Geometry check sheet. Reference: the model listing, model coordinates, mm. A direction names the side the tool comes from. Give positions to 0.01 mm unless a question says otherwise; leave off trailing zeros. Order: outer loops, then holes, each group sorted by start corner. A loop starts at its lowest first (then second) coordinate and runs counter-clockwise, first axis right, second up.
from build123d import *

# Parameters (mm, degrees)
SKETCH2_R           = 3.175
BOSS_EXTRUDE1_DEPTH = 1.57


with BuildPart() as part:
    # Sketch2 → Boss-Extrude1 (new body)
    with BuildSketch(Plane.XY.offset(5)):
        with BuildLine():
            Line((-16.920508995, 36.97485167), (-16.920508995, -35.724508995))
            Line((-16.920508995, -35.724508995), (-10.670508995, -35.724508995))
            Line((-10.670508995, -35.724508995), (-10.670508995, -24.224508995))
            Line((-10.670508995, -24.224508995), (10.670508995, -24.224508995))
            Line((10.670508995, -24.224508995), (10.670508995, -35.724508995))
            Line((10.670508995, -35.724508995), (16.920508995, -35.724508995))
            Line((16.920508995, -35.724508995), (16.920508995, 36.97485167))
            add(Edge.make_bspline(
                [(16.17485167, 37.720508995), (16.268017422, 37.720508995), (16.450238191, 37.688464247), (16.71855323, 37.51855323), (16.888464247, 37.250238191), (16.920508995, 37.068017422), (16.920508995, 36.97485167)],
                knots=[0, 0, 0, 0, 0.25, 0.5, 0.75, 1, 1, 1, 1], degree=3))
            Line((16.17485167, 37.720508995), (14.25, 37.720508995))
            ThreePointArc((14.25, 37.720508995), (11.718917637, 38.768917637), (10.670508995, 41.3))
            Line((10.670508995, 41.3), (10.670508995, 43.22485167))
            add(Edge.make_bspline(
                [(9.92485167, 43.970508995), (10.018017422, 43.970508995), (10.200238191, 43.938464247), (10.46855323, 43.76855323), (10.638464247, 43.500238191), (10.670508995, 43.318017422), (10.670508995, 43.22485167)],
                knots=[0, 0, 0, 0, 0.25, 0.5, 0.75, 1, 1, 1, 1], degree=3))
            Line((9.92485167, 43.970508995), (-9.92485167, 43.970508995))
            add(Edge.make_bspline(
                [(-10.670508995, 43.22485167), (-10.670508995, 43.318017422), (-10.638464247, 43.500238191), (-10.46855323, 43.76855323), (-10.200238191, 43.938464247), (-10.018017422, 43.970508995), (-9.92485167, 43.970508995)],
                knots=[0, 0, 0, 0, 0.25, 0.5, 0.75, 1, 1, 1, 1], degree=3))
            Line((-10.670508995, 43.22485167), (-10.670508995, 41.3))
            ThreePointArc((-10.670508995, 41.3), (-11.718917637, 38.768917637), (-14.25, 37.720508995))
            Line((-14.25, 37.720508995), (-16.17485167, 37.720508995))
            add(Edge.make_bspline(
                [(-16.920508995, 36.97485167), (-16.920508995, 37.068017422), (-16.888464247, 37.250238191), (-16.71855323, 37.51855323), (-16.450238191, 37.688464247), (-16.268017422, 37.720508995), (-16.17485167, 37.720508995)],
                knots=[0, 0, 0, 0, 0.25, 0.5, 0.75, 1, 1, 1, 1], degree=3))
        make_face()
        with Locations((0, -16.224508995)):
            Circle(SKETCH2_R, mode=Mode.SUBTRACT)
    extrude(amount=BOSS_EXTRUDE1_DEPTH)


solid = part.part
Item 1: Sectioned sample at B-B (y = -25.5). Enter the section's corners in (x, z).
Reported:
outline: (-16.92, 5) - (-10.67, 5) - (-10.67, 6.57) - (-16.92, 6.57) - close; (10.67, 5) - (16.92, 5) - (16.92, 6.57) - (10.67, 6.57) - close
Item 2: Sectioned sample at C-C (x = -12). Enter the section's corners in (y, z), and give its area (3 significant figures).
Reported:
outline: (-35.72, 5) - (38.52, 5) - (38.52, 6.57) - (-35.72, 6.57) - close
area: 117 mm2
Item 3: Sectioned sample at D-D (y = 39.5). Enter the section's corners in (x, z), and give its area (3 significant figures).
Reported:
outline: (-11.16, 5) - (11.16, 5) - (11.16, 6.57) - (-11.16, 6.57) - close
area: 35.0 mm2
Item 4: Gauge pin test, flat ends, axial feed: pin 1 (7.5 mm diameter, centred on x = 0, y = -16.22, fed in from +Z); pin 2 (0.8 mm diameter, centred on x = 0.5, z = 5.5, fed in from -Y); pin 3 (0.5 mm diameter, centred on x = 15, z = 5.5, fed in from +Y); pin 4 (0.8 mm diameter, centred on y = 42.5, z = 5.5, fed in from -X). Record the tip position at first contact, or that the pin passes through.
Reported:
pin 1: stops at z = 6.57
pin 2: stops at y = -24.22
pin 3: stops at y = 37.72
pin 4: stops at x = -10.67
Item 5: Set-up check for faces 4 (the flat face through (10.671, -30, 6)), 5 (the flat face through (16.921, 0, 6)), 6 (the flat face through (-10.671, 42, 6)), 7 (the flat face through (10.671, 42, 6)), 8 (the flat face through (0, 43.971, 6)): record each of +Z, -Z, +X, -X, +Y, -Y from which the full face is reachable in a straight line by a thin tool's end or side.
Reported:
face 4: +Z, -Z, -Y
face 5: +Z, -Z, +X, +Y, -Y
face 6: +Z, -Z, -X, +Y
face 7: +Z, -Z, +X, +Y
face 8: +Z, -Z, +X, -X, +Y
Item 6: Scan lines: L1, parallel to Y at x = 0, z = 5.45; L2, parallel to Y at x = 7.5, z = 5.1; L3, parallel to X at y = -25, z = 6.5. Record each from-to range of solid material in increasing order.
Reported:
L1: y = -24.22 to -19.4, -13.05 to 43.97
L2: y = -24.22 to 43.97
L3: x = -16.92 to -10.67, 10.67 to 16.92
Item 7: Draft check along X on faces 1 (the flat face through (-16.921, 1, 6)), 2 (the cylindrical face through (3.03, -15.27, 5.77)), 3 (the flat face through (15, 37.721, 6)). Enter one of: released by +X, released by -X, zero draft, split by the parting line, or undercut.
Reported:
face 1: released by -X
face 2: undercut
face 3: zero draft
Item 8: Sectioned sample at A-A (x = 0). Enter the section's corners in (y, z).
Reported:
outline: (-24.22, 5) - (-19.4, 5) - (-19.4, 6.57) - (-24.22, 6.57) - close; (-13.05, 5) - (43.97, 5) - (43.97, 6.57) - (-13.05, 6.57) - close
